Verification items for the finished model (mm, model axes). Face numbers are marked on the shaded views. A direction names the side the tool comes from. Coordinates: 2 decimals unless noted, no trailing zeros. Write each loop counter-clockwise with the first axis right and the second up, starting at its lowest first coordinate (ties: lowest second). Pieces come first, ordered by that corner, then holes. Notation, with made-up numbers: (76, 33) - (86, 33) arc R27 ccw to (86, 55) - close; hole circle Ø10 at (8, -37.75). An arc over 180 degrees is marked (long way). Answer as CSV lines item,"result". Start each with the question number.
Autodesk Inventor part; units mm, degrees
ref_plane "YZ Plane" through (0, 0, 0) normal (1, 0, 0) x (0, 1, 0)
ref_plane "XZ Plane" through (0, 0, 0) normal (0, 1, 0) x (-1, 0, 0)
ref_plane "XY Plane" through (0, 0, 0) normal (0, 0, 1) x (1, 0, 0)
sketch "Sketch1" plane through (0, 0, 0) normal (0, 0, 1) x (1, 0, 0)
  circle A0 centre (0, 0) radius 5.588
  circle A1 centre (0, 0) radius 11.303
  dimension "d0" = 11.176
  dimension "d1" = 22.606
extrude "Extrusion1" add sketch "Sketch1" along normal mid plane 1.27
sketch "Sketch2" plane through (0, 0, 0.635) normal (0, 0, 1) x (1, 0, 0)
  circle A0 centre (0, 0) radius 11.303
  circle A1 centre (0, 0) radius 9.017
  line L0 (0, 0) -> (-7.9924, 7.9924) construction
  line L1 (0, 0) -> (-16.0053, 0) construction
  line L2 (-3.0848, 8.4729) -> (-2.2451, 2.2451)
  line L3 (-2.2451, 2.2451) -> (-8.4729, 3.0848)
  dimension "d4" = 2.286
  dimension "d5" = 45
  dimension "d6" = 3.175
  dimension "d7" = 7.62
extrude "Extrusion2" cut sketch "Sketch2" against normal through all contours L2 L3 A1 picked at (-6.1075, 3.3917)
pattern_circular "Circular Pattern1" count 4 over 360 about axis through (0, 0, -10) along (0, 0, 1) of "Extrusion2"
sketch "Sketch3" plane through (0, 0, 0.635) normal (0, 0, 1) x (1, 0, 0)
  line L0 (2.6087, 4.9417) -> (3.0848, 8.4729)
  arc A0 (8.4729, 3.0848) -> (3.0848, 8.4729) centre (0, 0) ccw
  line L1 (8.4729, 3.0848) -> (4.9417, 2.6087)
  arc A1 (4.9417, -2.6087) -> (4.9417, 2.6087) centre (0, 0) ccw
  line L2 (4.9417, -2.6087) -> (8.4729, -3.0848)
  arc A2 (3.0848, -8.4729) -> (8.4729, -3.0848) centre (0, 0) ccw
  line L3 (3.0848, -8.4729) -> (2.6087, -4.9417)
  arc A3 (-2.6087, -4.9417) -> (2.6087, -4.9417) centre (0, 0) ccw
  line L4 (-2.6087, -4.9417) -> (-3.0848, -8.4729)
  arc A4 (-8.4729, -3.0848) -> (-3.0848, -8.4729) centre (0, 0) ccw
  line L5 (-8.4729, -3.0848) -> (-4.9417, -2.6087)
  arc A5 (-4.9417, 2.6087) -> (-4.9417, -2.6087) centre (0, 0) ccw
  line L6 (-4.9417, 2.6087) -> (-8.4729, 3.0848)
  arc A6 (-3.0848, 8.4729) -> (-8.4729, 3.0848) centre (0, 0) ccw
  line L7 (-3.0848, 8.4729) -> (-2.6087, 4.9417)
  arc A7 (2.6087, 4.9417) -> (-2.6087, 4.9417) centre (0, 0) ccw
  circle A8 centre (0, 0) radius 11.303
  line L8 (-3.0848, -8.4729) -> (-3.3959, -10.7808)
  circle A9 centre (0, 0) radius 11.303
  line L9 (3.0848, -8.4729) -> (3.3959, -10.7808)
  line L10 (-2.6087, -4.9417) -> (-3.0848, -8.4729)
  line L11 (3.0848, -8.4729) -> (2.6087, -4.9417)
extrude "Extrusion3" cut sketch "Sketch3" against normal through all contours L9 A8 L8 L4 A3 L3
fillet "Fillet1" radius 1.27 6 edges at (-8.4729, -3.0848, 0) (8.4729, -3.0848, 0) (8.4729, 3.0848, 0) (3.0848, 8.4729, 0) (-3.0848, 8.4729, 0) (-8.4729, 3.0848, 0)
fillet "Fillet1" radius 0.635 10 edges at (-4.9417, -2.6087, 0) (-4.9417, 2.6087, 0) (-2.6087, 4.9417, 0) (2.6087, 4.9417, 0) (4.9417, 2.6087, 0) (4.9417, -2.6087, 0) (-3.0848, -8.4729, 0) (-3.3959, -10.7808, 0) (3.3959, -10.7808, 0) (3.0848, -8.4729, 0)
properties part number "External Klipring for 500 shaft (am-0206)" material "Steel, Carbon"
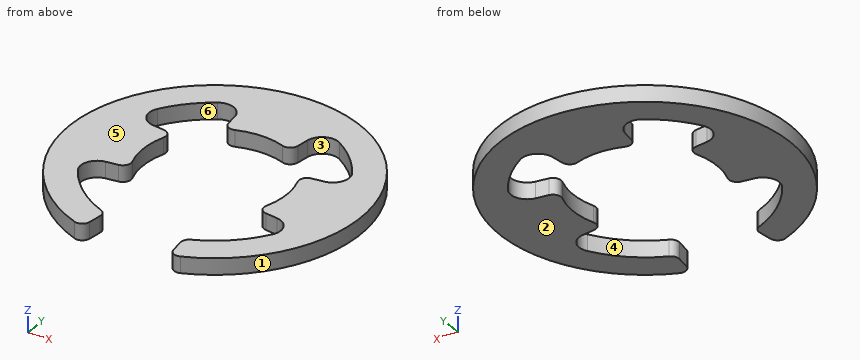
1. Cross-section at C-C (y = -0.25). Record the cut outline in (x, z) (3 decimals).
2. Draft check along X on the marked faces 1, 2, 3 and 4. Enter one of: pulls with the +X half, pulls with the -X half, needs draft (parallel to the pull), parting line crosses it, or undercut.
3. Scan lines: line 1 along Y through (x, z) = (7, 0.2); line 2 along Y through (x, z) = (7.5, -0.4); line 3 along X through (y, z) = (-7.75, 0.05). Record each from-to range of solid material in increasing order. Write a range as from..to.
4. Cross-section at D-D (x = 0). Record the cut outline in (y, z) (3 decimals), and give its area (3 significant figures).
5. Access from +Z, -Z, +X, -X, +Y, -Y to the whole of each face (thin tool, end or side, straight path). Record for the marked faces 5 and 6.
6. Cross-section at A-A (y = -5.75). Record the cut outline in (x, z) (3 decimals), and give its area (3 significant figures).
Completed:
1,outline,"(-11.3, -0.635) - (-5.582, -0.635) - (-5.582, 0.635) - (-11.3, 0.635) - close; (5.582, -0.635) - (11.3, -0.635) - (11.3, 0.635) - (5.582, 0.635) - close"
2,face 1,"parting line crosses it"
2,face 2,"needs draft"
2,face 3,"undercut"
2,face 4,"undercut"
3,line 1,"y = -8.87..-5.68, -2.92..2.92, 5.68..8.87"
3,line 2,"y = -8.46..-5.01, -3.25..3.25, 5.01..8.46"
3,line 3,"x = -8.23..-4.61, 4.61..8.23"
4,outline,"(5.588, -0.635) - (11.303, -0.635) - (11.303, 0.635) - (5.588, 0.635) - close"
4,area,"7.26 mm2"
5,face 5,"+Z, +X, -X, +Y, -Y"
5,face 6,"+Z, -Z"
6,outline,"(-9.731, -0.635) - (-6.946, -0.635) - (-6.946, 0.635) - (-9.731, 0.635) - close; (6.946, -0.635) - (9.731, -0.635) - (9.731, 0.635) - (6.946, 0.635) - close"
6,area,"7.07 mm2"
